For this review, take the finished solid that the model builds, in its own axes (mm). A direction names the side the tool comes from. Round coordinates to 2 decimals unless told otherwise and drop trailing zeros. Order: outer loops, then holes, each group sorted by start corner. A loop starts at its lowest first (then second) coordinate and runs counter-clockwise, first axis right, second up. Notation, with made-up numbers: M 21,69 L 61,69 A12 ccw 61,73 Z; hole C 88.5,39.5 d5. An arc over 180 degrees is marked long. Put each result on its own line as item: value.
from build123d import *

# Parameters (mm, degrees)
BOSS_EXTRUDE1_DEPTH = 6


with BuildPart() as part:
    # Sketch1 → Boss-Extrude1 (new body)
    with BuildSketch(Plane(origin=(0, 0, 0), x_dir=(1, 0, 0), z_dir=(0, 1, 0))):
        with BuildLine():
            Line((0, 8.467832856), (0, -3.532167144))
            ThreePointArc((0, -3.532167144), (-1.915343114, -4.849607871), (-2.460583977, -2.589762364))
            ThreePointArc((-2.460583977, -2.589762364), (-1.803306785, -1.595054715), (-1.463898856, -0.452137887))
            Line((-1.463898856, -0.452137887), (-2.5, 0.664908658))
            Line((-2.5, 0.664908658), (-2.5, 6.634329976))
            Line((-2.5, 6.634329976), (-0.586152098, 8.409493247))
            Line((-0.586152098, 8.409493247), (0, 8.467832856))
        make_face()
    extrude(amount=BOSS_EXTRUDE1_DEPTH)


solid = part.part
(1) Add section C-C on x = -1.75. Give the boundary of the cut face in (y, z).
A:
outline: M 0,-7.33 L 6,-7.33 L 6,0.14 L 0,0.14 Z; M 0,1.48 L 6,1.48 L 6,4.9 L 0,4.9 Z
(2) For faces 1 (the face through (-2.5, 3, -4)), 2 (the face through (-1.81, 2.96, 1.61)), 3 (the face through (-1, 0, -2)), list the 3-axis set-ups (+Z, -Z, +X, -X, +Y, -Y) from which the entire face can be reached by the end or side of a thin tool; tool diameter is ignored.
A:
face 1: -Z, -X, +Y, -Y
face 2: -X, +Y, -Y
face 3: +Z, -Z, +X, -X, -Y
(3) Add section A-A on x = -2.3. Give the boundary of the cut face in (y, z).
A:
outline: M 0,-6.82 L 6,-6.82 L 6,-0.45 L 0,-0.45 Z; M 0,2.4 L 6,2.4 L 6,4.63 L 0,4.63 Z
(4) Draft analysis for pull direction Z (two halves, no side actions). For faces 4 (the face through (-1.975, 2.958, -0.099)), 5 (the face through (-1.556, 2.958, -7.509)), 6 (the face through (0, 3, -3)), state which applies: released by +Z, released by -Z, zero draft, split by the parting line, or undercut.
A:
face 4: undercut
face 5: released by -Z
face 6: zero draft
(5) Add section B-B on y = 1.95. Give the boundary of the cut face in (x, z), then the cut area to 3 significant figures.
A:
outline: M -2.5,-6.63 L -0.59,-8.41 L 0,-8.47 L 0,3.53 A1.41 ccw long -2.46,2.59 A4.05 cw -1.46,0.45 L -2.5,-0.66 Z
area: 29.5 mm2
(6) Insertion check: pin 1 Ø3 at (y, z) = (4.5, -3.5) entering from -X. The pin has a flat end and moves straight along its axis. Give the tip position at first contact, or say it passes through.
A:
pin 1: stops at x = -2.5
(7) Add section D-D on z = -4.5. Give the boundary of the cut face in (x, y), then the cut area to 3 significant figures.
A:
outline: M -2.5,0 L 0,0 L 0,6 L -2.5,6 Z
area: 15.0 mm2
(8) To check wall thickness, follow L1, parallel to Z at x = -2.35, y = 4.85; L2, parallel to X at y = 2.9, z = -2.5; L3, parallel to Z at x = -2, y = 1.55. State the ranges of each line that lie inside material, in increasing order.
A:
L1: z = -6.77 to -0.5, 2.46 to 4.58
L2: x = -2.5 to 0
L3: z = -7.1 to -0.13, 1.97 to 4.81
